Design review of the part shown in the three views and the two pictorial views. Dimensions are in mm from the part's minimum x, y and z. A direction names the side the tool comes from. Round coordinates to 2 decimals unless told otherwise and drop trailing zeros. Order: outer loops, then holes, each group sorted by start corner. A loop starts at its lowest first (then second) coordinate and runs counter-clockwise, first axis right, second up. Notation, with made-up numbers: M -36,71 L -30,71 A23 cw -30,97 Z; hole C -39,66.5 d6. An arc over 180 degrees is marked long. Write each question's results on one line, items separated by ' | '. Start each with the question number.
Item 1: Take a section at B-B, the plane z = 1.5. Write out the cut boundary in (x, y).
Item 2: The part is to be moulded in two halves that separate along Y. For the marked faces 4, 5 and 6, say which applies: +Y half, -Y half, draft (parallel to the pull), parting line (faces both ways), or undercut.
Item 3: Wall thickness on line 1 (Y direction, x = 3.3, z = 8.75); line 2 (Z direction, x = 2.55, y = 0.9); line 3 (Z direction, x = 3.15, y = 3.2): over which ranges is each line inside the solid? List them lowest first. Write a range as [from, to].
Item 4: Machinability: for the marked faces 1, 2 and 3, which of the approach directions +Z, -Z, +X, -X, +Y, -Y give a long, thin tool a straight path to every point of the face, cutting with its end or side? Answer none if there is none.
Item 5: Take a section at A-A, the plane z = 7.25. Write out the cut boundary in (x, y).
Item 6: Clearance check with flat-ended pins moving along their axes: pin 1 (3 mm diameter, centred on x = 2, y = 3.5, fed in from -Z); pin 2 (1 mm diameter, centred on x = 3, z = 2, fed in from +Y). State where each tip first meets the part, or that it passes through.
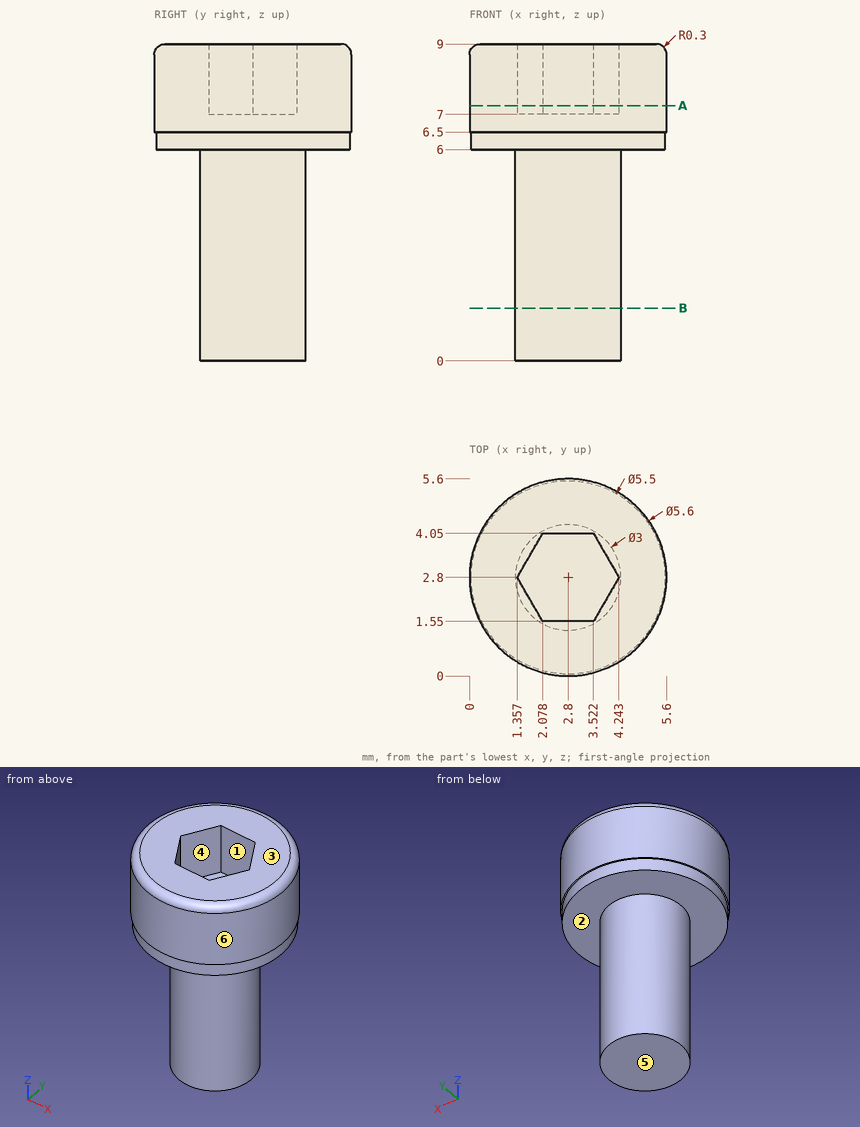
Results list:
1) outline: C 2.8,2.8 d3
2) face 4: undercut | face 5: draft | face 6: parting line
3) line 1: [0.05, 1.55], [4.05, 5.55] | line 2: [6, 9] | line 3: [0, 7]
4) face 1: +Z | face 2: -Z | face 3: +Z, +X, -X, +Y, -Y
5) outline: C 2.8,2.8 d5.6; hole M 1.36,2.8 L 2.08,1.55 L 3.52,1.55 L 4.24,2.8 L 3.52,4.05 L 2.08,4.05 Z
6) pin 1: z = 0 | pin 2: y = 4.3
